Verification items for the finished model (mm, model axes). Round coordinates to 2 decimals unless told otherwise and drop trailing zeros. Order: outer loops, then holes, each group sorted by start corner. A loop starts at its lowest first (then second) coordinate and runs counter-clockwise, first axis right, second up. Notation, with made-up numbers: M -8,57 L 1,57 A16 cw 1,82 Z; hole C -18.5,29 d5. An arc over 180 degrees is marked long. Write item = value, one per line. Start each with the question number.
from build123d import *

# Parameters (mm, degrees)
F0_R     = 1.5
F0_R_2   = 11.3
F1_DEPTH = 4


with BuildPart() as f1:
    # F0 (on Top) → F1 (new body)
    with BuildSketch(Plane.XY):
        with BuildLine():
            Line((-20.590143, 17.982571), (-27.672114, 1.586057))
            ThreePointArc((-27.672114, 1.586057), (-28, 0), (-27.672114, -1.586057))
            Line((-27.672114, -1.586057), (-20.590143, -17.982571))
            ThreePointArc((-20.590143, -17.982571), (-18.746556, -20.178089), (-16, -21))
            Line((-16, -21), (16, -21))
            ThreePointArc((16, -21), (18.746556, -20.178089), (20.590143, -17.982571))
            Line((20.590143, -17.982571), (27.672114, -1.586057))
            ThreePointArc((27.672114, -1.586057), (28, 0), (27.672114, 1.586057))
            Line((27.672114, 1.586057), (20.590143, 17.982571))
            ThreePointArc((20.590143, 17.982571), (18.746556, 20.178089), (16, 21))
            Line((16, 21), (-16, 21))
            ThreePointArc((-16, 21), (-18.746556, 20.178089), (-20.590143, 17.982571))
        make_face()
        with Locations((-15.5, -15.5)):
            Circle(F0_R, mode=Mode.SUBTRACT)
        with Locations((15.5, -15.5)):
            Circle(F0_R, mode=Mode.SUBTRACT)
        with Locations((-24, 0)):
            Circle(F0_R, mode=Mode.SUBTRACT)
        with Locations((-15.5, 15.5)):
            Circle(F0_R, mode=Mode.SUBTRACT)
        Circle(F0_R_2, mode=Mode.SUBTRACT)
        with Locations((24, 0)):
            Circle(F0_R, mode=Mode.SUBTRACT)
        with Locations((15.5, 15.5)):
            Circle(F0_R, mode=Mode.SUBTRACT)
    extrude(amount=F1_DEPTH)


solid = f1.part
1) Cross-section at A-A, the plane x = 0. Enter the section's corners in (y, z), then the cut area to 3 significant figures.
2) Scan lines: probe 1 along Y at (x, z) = (15, 0.65); probe 2 along Y at (x, z) = (-15.5, 1.45); probe 3 along Y at (x, z) = (-0.5, 3.2). Record each from-to range of solid material in increasing order.
3) Cross-section at D-D, the plane x = -24. Enter the section's corners in (y, z), then the cut area to 3 significant figures.
4) Cross-section at C-C, the plane y = 15.5. Enter the section's corners in (x, z).
5) Cross-section at B-B, the plane z = 1.8. Enter the section's corners in (x, y), then the cut area to 3 significant figures.
6) Release check for a two-part mould opening along X. For faces 1 (the cylindrical face through (22.5, 0.07, 1.97)), 2 (the cylindrical face through (-19, 20, 2)), 3 (the flat face through (24.18, 9.67, 1.97)), 4 (the cylindrical face through (-17, 15.57, 1.97)) record: pulls with the +X half, pulls with the -X half, needs draft (parallel to the pull), parting line crosses it, or undercut.
Geometry results:
q1.outline = M -21,0 L -11.3,0 L -11.3,4 L -21,4 Z; M 11.3,0 L 21,0 L 21,4 L 11.3,4 Z
q1.area = 77.6 mm^2
q2.probe_1 = -21 to -16.91, -14.09 to 14.09, 16.91 to 21
q2.probe_2 = -21 to -17, -14 to 14, 17 to 21
q2.probe_3 = -21 to -11.29, 11.29 to 21
q3.outline = M -10.09,0 L -1.5,0 L -1.5,4 L -10.09,4 Z; M 1.5,0 L 10.09,0 L 10.09,4 L 1.5,4 Z
q3.area = 68.7 mm^2
q4.outline = M -21.66,0 L -17,0 L -17,4 L -21.66,4 Z; M -14,0 L 14,0 L 14,4 L -14,4 Z; M 17,0 L 21.66,0 L 21.66,4 L 17,4 Z
q5.outline = M -27.67,-1.59 L -20.59,-17.98 A5 ccw -16,-21 L 16,-21 A5 ccw 20.59,-17.98 L 27.67,-1.59 A4 ccw 27.67,1.59 L 20.59,17.98 A5 ccw 16,21 L -16,21 A5 ccw -20.59,17.98 L -27.67,1.59 A4 ccw Z; hole C -24,0 d3; hole C -15.5,-15.5 d3; hole C -15.5,15.5 d3; hole C 0,0 d22.6; hole C 15.5,-15.5 d3; hole C 15.5,15.5 d3; hole C 24,0 d3
q5.area = 1,550 mm^2
q6.face_1 = undercut
q6.face_2 = pulls with the -X half
q6.face_3 = pulls with the +X half
q6.face_4 = undercut
